The listing builds one solid part. Answer for the finished solid, in the listing's coordinates (mm). A direction names the side the tool comes from. Coordinates: 2 decimals unless noted, no trailing zeros. Write each loop counter-clockwise with the first axis right and the second up, starting at its lowest first coordinate (ties: lowest second). Pieces come first, ordered by that corner, then holes. Notation, with made-up numbers: M 19.25,50 L 62.25,50 A35 cw 62.25,85 Z; hole C -2.5,28.5 d8. An arc over 180 degrees is marked long. Answer as CSV lines item,"result".
Autodesk Inventor part; units mm, degrees
ref_plane "YZ Plane" through (0, 0, 0) normal (1, 0, 0) x (0, 1, 0)
ref_plane "XZ Plane" through (0, 0, 0) normal (0, 1, 0) x (-1, 0, 0)
ref_plane "XY Plane" through (0, 0, 0) normal (0, 0, 1) x (1, 0, 0)
sketch "Sketch1" plane through (0, 0, 0) normal (0, 0, 1) x (1, 0, 0)
  circle A0 centre (0, 0) radius 33
  circle A1 centre (0, 0) radius 16.5
  circle A2 centre (25, 0) radius 3.5
  circle A3 centre (-12.5, 21.6506) radius 3.5
  circle A4 centre (-12.5, -21.6506) radius 3.5
  dimension "d0" = 66
  dimension "d1" = 33
  dimension "d2" = 7
  dimension "d3" = 25
  dimension "d6" = 360
extrude "Extrusion1" add sketch "Sketch1" along normal blind 35
sketch "Sketch3" plane through (0, 0, 35) normal (0, 0, 1) x (1, 0, 0)
  circle A0 centre (3.125, 0) radius 53
  circle A1 centre (0, 0) radius 10
  circle A2 centre (26.625, -40.7032) radius 3.15
  circle A3 centre (18.75, 0) radius 5.5
  circle A4 centre (50.125, 0) radius 3.15
  circle A5 centre (26.625, 40.7032) radius 3.15
  circle A6 centre (3.125, -47) radius 3.15
  circle A7 centre (3.125, 47) radius 3.15
  circle A8 centre (-43.875, 0) radius 3.15
  line L0 (3.125, 0) -> (3.125, 47)
  line L1 (3.125, 0) -> (26.625, 40.7032)
  line L2 (3.125, 0) -> (50.125, 0)
  line L3 (26.625, -40.7032) -> (3.125, 0)
  line L4 (3.125, 0) -> (3.125, -47)
  line L5 (3.125, 0) -> (-43.875, 0)
  circle A9 centre (0, 0) radius 33
  point P0 (0, 0)
  dimension "d19" = 106
  dimension "d20" = 6.3
  dimension "d21" = 6.3
  dimension "d22" = 6.3
  dimension "d23" = 6.3
  dimension "d24" = 6.3
  dimension "d25" = 6.3
  dimension "d27" = 20
  dimension "d28" = 18.75
  dimension "d35" = 30
  dimension "d36" = 30
  dimension "d37" = 3.125
  dimension "d38" = 11
  dimension "d41" = 47
  dimension "d44" = 47
  dimension "d45" = 47
  dimension "d46" = 47
  dimension "d47" = 47
  dimension "d48" = 47
extrude "Extrusion4" add sketch "Sketch3" against normal blind 10
sketch "Sketch4" plane through (3.125, 0, 35) normal (0, 0, 1) x (1, 0, 0)
  circle A0 centre (18.75, 0) radius 7.5
  point P0 (-3.125, 0)
  dimension "d49" = 15
  dimension "d50" = 21.875
extrude "Extrusion5" cut sketch "Sketch4" against normal blind 5
sketch "Sketch5" plane through (3.125, 0, 35) normal (0, 0, 1) x (1, 0, 0)
  circle A0 centre (21.875, 0) radius 3.5
  circle A1 centre (21.875, 0) radius 3.5
  circle A2 centre (21.875, 0) radius 12.5
  circle A3 centre (-15.625, 21.6506) radius 12.5
  circle A4 centre (-15.625, -21.6506) radius 12.5
  point P0 (-3.125, 0)
  dimension "d53" = 25
  dimension "d56" = 360
extrude "Extrusion6" cut sketch "Sketch5" against normal blind 8 contours A0 | A2 | A3 | A4
properties part number "AC10" material "ABS Plastic"
Q1. Find section A-A (y = 0). Give the vertices of the cut face in (x, z) (3 decimals).
Output:
outline,"M -49.875,25 L -47.025,25 L -47.025,35 L -49.875,35 Z; M -40.725,25 L -33,25 L -33,0 L -16.5,0 L -16.5,35 L -40.725,35 Z; M 16.5,0 L 21.5,0 L 21.5,27 L 16.5,27 Z; M 28.5,0 L 33,0 L 33,25 L 46.975,25 L 46.975,35 L 37.5,35 L 37.5,27 L 28.5,27 Z; M 53.275,25 L 56.125,25 L 56.125,35 L 53.275,35 Z"
Q2. For faces 1 (the flat face through (-15.5, -24.3, 27)), 2 (the flat face through (26, -23, 25)), 3 (the cylindrical face through (26.215, 43.826, 30.07)), determine the directions among +Z, -Z, +X, -X, +Y, -Y from which every point of the face is accessible in a straight line to the end or side of a thin tool.
Output:
face 1,"+Z"
face 2,"-Z"
face 3,"+Z, -Z"
Q3. Flat-ended cylindrical pins translate along their axes: pin 1 Ø20 at (x, y) = (25, 0) entering from +Z; pin 2 Ø1.5 at (y, z) = (4, 22.5) entering from +X; pin 3 Ø3 at (x, z) = (-17, 6.5) entering from +Y; pin 4 Ø5 at (x, y) = (3.125, -47) entering from +Z. Find the tip coordinate at first contact, or state that the pin passes through.
Output:
pin 1,"z = 27"
pin 2,"x = 32.84"
pin 3,"y = 29.13"
pin 4,"through"
Q4. Straight lines are drawn through the part: line 1 (Z direction, x = -4.5, y = 41); line 2 (Z direction, x = -20.5, y = 14.5); line 3 (X direction, y = 14.5, z = 17.5). For each, find the intervals that lie inside material, in ascending order.
Output:
line 1,"25 to 35"
line 2,"0 to 27"
line 3,"-29.64 to -7.87, 7.87 to 29.64"
Q5. Find section C-C (y = -47). Give the vertices of the cut face in (x, z) (3 decimals).
Output:
outline,"M -21.37,25 L -0.025,25 L -0.025,35 L -21.37,35 Z; M 6.275,25 L 27.62,25 L 27.62,35 L 6.275,35 Z"
Q6. Find section D-D (z = 22). Give the vertices of the cut face in (x, y).
Output:
outline,"C 0,0 d66; hole C 0,0 d33; hole C -12.5,-21.65 d7; hole C -12.5,21.65 d7; hole C 25,0 d7"
Q7. Find section B-B (x = 9.5). Give the vertices of the cut face in (y, z).
Output:
outline,"M -52.62,25 L -31.6,25 L -31.6,0 L -13.49,0 L -13.49,35 L -52.62,35 Z; M 13.49,0 L 31.6,0 L 31.6,25 L 52.62,25 L 52.62,35 L 13.49,35 Z"
Q8. The mould has two halves that part along Y. Classify faces 4 (the cylindrical face through (-19.128, -32.248, 31.056)), 5 (the flat face through (14, -11, 35)), 6 (the cylindrical face through (30.5, 12.6, 12.3)): pulls with the +Y half, pulls with the -Y half, needs draft (parallel to the pull), parting line crosses it, or undercut.
Output:
face 4,"undercut"
face 5,"needs draft"
face 6,"parting line crosses it"
